Autodesk Inventor part; units mm, degrees
ref_plane "Work Plane1" through (0, 0, -15) normal (0, 0, 1) x (1, 0, 0)
ref_plane "YZ Plane" through (0, 0, 0) normal (1, 0, 0) x (0, 1, 0)
ref_plane "XZ Plane" through (0, 0, 0) normal (0, 1, 0) x (-1, 0, 0)
sketch "Sketch1" plane through (0, 0, 0) normal (0, 0, 1) x (1, 0, 0)
  line L0 (0, 0) -> (25, 0)
  line L1 (25, 0) -> (25, 40)
  line L2 (25, 40) -> (0, 40)
  line L3 (0, 40) -> (0, 0)
  dimension "d1" = 25
  dimension "d2" = 40
  dimension "d3" = 25
extrude "Extrusion1" add sketch "Sketch1" against normal blind 30
sketch "Sketch2" plane through (25, 0, 0) normal (1, 0, 0) x (0, 0, -1)
  line L0 (0, 0) -> (30, 0)
  circle A0 centre (15, 6.56) radius 2.46
extrude "Extrusion2" cut sketch "Sketch2" against normal blind 30
sketch "Sketch3" plane through (0, 0, 0) normal (-1, 0, 0) x (0, 0, 1)
  line L0 (0, 0) -> (-30, 0)
  line L1 (-25.05, 0) -> (-4.95, 0)
  line L2 (-4.95, 0) -> (-4.95, 33.12)
  line L3 (-4.95, 33.12) -> (-25.05, 33.12)
  line L4 (-25.05, 33.12) -> (-25.05, 0)
  dimension "d11" = 20.1
extrude "Extrusion3" cut sketch "Sketch3" against normal blind 20
sketch "Sketch4" plane through (0, 0, 0) normal (0, -1, 0) x (1, 0, 0)
  line L0 (20, -4.95) -> (20, -25.05)
  line L1 (20, -15) -> (25, -15)
  line L2 (25, 0) -> (25, -30)
  line L3 (20, -8.025) -> (25, -8.025)
  line L4 (25, -8.025) -> (25, -21.975)
  line L5 (25, -21.975) -> (20, -21.975)
  line L6 (20, -21.975) -> (20, -8.025)
  line L7 (20, -8.025) -> (25, -21.975) construction
  line L8 (25, -8.025) -> (20, -21.975) construction
  line L9 (25, -12.54) -> (25, -17.46)
  point P0 (0, 0)
  point P1 (22.5, -15)
  dimension "d14" = 13.95
extrude "Extrusion4" add sketch "Sketch4" along normal blind 15
sketch "Sketch5" plane through (20, 0, 0) normal (-1, 0, 0) x (0, 0, 1)
  circle A0 centre (-15, 6.56) radius 2.46
  circle A1 centre (-15, 6.56) radius 4.7025
  circle A2 centre (-15, 6.56) radius 2.46
  circle A3 centre (-15, 6.56) radius 2.46
  point P0 (0, 0)
  dimension "d17" = 9.405
extrude "Extrusion5" cut sketch "Sketch5" against normal blind 2.1
sketch "Sketch6" plane through (25, 0, 0) normal (1, 0, 0) x (0, 0, -1)
  circle A0 centre (15, 6.56) radius 4.7025
  line L0 (15, 6.56) -> (15, 23.56)
  circle A1 centre (15, 23.56) radius 2.46
  point P0 (0, 0)
  dimension "d20" = 17
  dimension "d21" = 4.92
extrude "Extrusion6" cut sketch "Sketch6" against normal blind 10 contours A1
sketch "Sketch7" plane through (20, 0, 0) normal (-1, 0, 0) x (0, 0, 1)
  circle A0 centre (-15, 23.56) radius 2.46
  circle A1 centre (-15, 23.56) radius 4.7025
  point P0 (0, 0)
  dimension "d24" = 9.405
extrude "Extrusion7" cut sketch "Sketch7" against normal blind 2.1
sketch "Sketch9" plane through (25, 0, 0) normal (1, 0, 0) x (0, 0, -1)
  circle A0 centre (15, 6.56) radius 2.46
  circle A1 centre (15, 6.56) radius 2.46
  circle A2 centre (15, 23.56) radius 2.46
  circle A3 centre (15, 23.56) radius 2.46
  line L0 (30, 40) -> (30, 0)
  line L1 (30, 0) -> (30, 40)
  line L2 (30, 40) -> (0, 40)
  line L3 (0, 40) -> (0, 0)
  line L4 (0, 0) -> (8.025, 0)
  line L5 (21.975, 0) -> (21.975, -15)
  line L6 (21.975, -15) -> (8.025, -15)
  line L7 (8.025, -15) -> (8.025, 0)
  line L8 (0, 0) -> (8.025, 0)
  line L9 (21.975, 0) -> (30, 0)
extrude "Extrusion8" add sketch "Sketch9" along normal blind 5
sketch "Sketch10" plane through (0, 40, 0) normal (0, 1, 0) x (1, 0, 0)
  line L0 (0, 30) -> (30, 30)
  line L1 (30, 0) -> (0, 0)
  line L2 (0, 30) -> (30, 30)
  line L3 (30, 30) -> (30, 0)
  line L4 (30, 0) -> (0, 0)
  line L5 (0, 0) -> (0, 30)
extrude "Extrusion9" add sketch "Sketch10" along normal blind 30
sketch "Sketch12" plane through (30, 0, 0) normal (1, 0, 0) x (0, 0, -1)
  circle A0 centre (15, 6.56) radius 2.46
  line L0 (15, 6.56) -> (15, 15.06)
  circle A1 centre (15, 15.06) radius 2.525
  point P0 (0, 0)
  dimension "d31" = 8.5
  dimension "d33" = 5.05
extrude "Extrusion10" cut sketch "Sketch12" against normal blind 30 contours A1
sketch "Sketch14" plane through (0, 0, 0) normal (0, 0, 1) x (1, 0, 0)
  line L0 (30, 70) -> (0, 70)
  line L1 (0, 100) -> (-8, 100)
  line L2 (30, 0) -> (30, 70)
  line L3 (30, 118) -> (30, 70)
  line L4 (30, 105) -> (30, 100)
  line L5 (0, 70) -> (30, 70)
  line L6 (0, 70) -> (0, 100)
  line L7 (15, 136) -> (30, 118)
  line L8 (-8, 136) -> (15, 136)
  line L9 (-8, 100) -> (-8, 136)
  point P0 (0, 0)
  dimension "d47" = 30
extrude "Extrusion12" add sketch "Sketch14" against normal blind 30
sketch "Sketch15" plane through (0, 0, -25.05) normal (-1, 0, 0) x (0, 0, 1)
  line L0 (0, 33.12) -> (20.1, 33.12)
  line L1 (20.1, 33.12) -> (20.1, 0)
  line L2 (0, 33.12) -> (20.1, 33.12)
  line L3 (20.1, 33.12) -> (20.1, 31.1)
  line L4 (20.1, 31.1) -> (0, 31.1)
  line L5 (0, 31.1) -> (0, 33.12)
  point P0 (25.05, 0)
  dimension "d57" = 2.02
extrude "Extrusion13" add sketch "Sketch15" against normal blind 20
sketch "Sketch23" plane through (0, 0, 0) normal (0, 0, 1) x (1, 0, 0)
  line L0 (0, 100) -> (-8, 100)
  line L1 (-8, 136) -> (15, 136)
  line L2 (-8, 136) -> (15, 136)
  line L3 (30, 118) -> (15, 136)
  line L4 (15, 136) -> (30, 118)
  line L5 (30, 118) -> (30, 93)
  line L6 (30, 0) -> (30, 118)
  line L7 (30, 93) -> (0, 93)
  line L8 (0, 93) -> (0, 100)
  line L9 (-8, 100) -> (0, 100)
  line L10 (15, 136) -> (-8, 136)
  line L11 (-8, 136) -> (-8, 100)
  point P0 (0, 0)
  point P1 (-2, 102)
  point P2 (4, 118)
  point P3 (-2, 134)
  dimension "d85" = 25
extrude "Extrusion14" add sketch "Sketch23" along normal blind 15
ref_plane "Work Plane1" through (0, 0, -15) normal (0, 0, 1) x (1, 0, 0)
mirror "Mirror1" about plane through (0, 0, -15) normal (0, 0, 1) of "Extrusion14"
sketch "Sketch28" plane through (-8, 136, 15) normal (0, 1, 0) x (1, 0, 0)
  line L0 (0, 60) -> (0, 0)
  line L1 (0, 30) -> (0, 5)
  line L2 (0, 5) -> (5, 5)
  line L3 (5, 5) -> (5, 55)
  line L4 (5, 55) -> (0, 55)
  line L5 (0, 55) -> (0, 30)
  line L6 (0, 55) -> (5, 30)
  line L7 (5, 30) -> (0, 5)
  point P0 (8, 15)
  dimension "d100" = 25
  dimension "d101" = 5
  dimension "d102" = 50
extrude "Extrusion17" cut sketch "Sketch28" against normal through all contours L6 L7 L0
properties part number "orien_b_45mm"
For this review, take the finished solid that the model builds, in its own axes (mm). A direction names the side the tool comes from. Coordinates: 2 decimals unless noted, no trailing zeros. Order: outer loops, then holes, each group sorted by start corner. A loop starts at its lowest first (then second) coordinate and runs counter-clockwise, first axis right, second up. Notation, with made-up numbers: (-25, 80.5) -> (-4, 80.5) arc R35 cw to (-4, 119.5) -> close; hole circle Ø5 at (62, 83.25). An arc over 180 degrees is marked (long way). Answer as CSV lines item,"result".
Q1. For faces 5 (the face through (10, 16, -25.05)), 6 (the face through (15, 47, 0)), 7 (the face through (21.035, 7.973, -10.515)), 8 (the face through (-2, 100, -15)), 9 (the face through (15, 47, -30)), list the 3-axis set-ups (+Z, -Z, +X, -X, +Y, -Y) from which the entire face can be reached by the end or side of a thin tool; tool diameter is ignored.
Model answer:
face 5,"-X, -Y"
face 6,"+Z, +X, -X, -Y"
face 7,"-X"
face 8,"+Z, -Z, -X, -Y"
face 9,"-Z, +X, -X, -Y"
Q2. Wall thickness on line 1 along Z through (x, y) = (3.5, 9); line 2 along Y through (x, z) = (27, -15) (3 decimals); line 3 along Y through (x, z) = (25, -15) (3 decimals): over which ranges is each line inside the solid? List them lowest first. Write a range as [from, to].
Model answer:
line 1,"z = [-30, -25.05], [-4.95, 0]"
line 2,"y = [-15, 4.1], [9.02, 12.535], [17.585, 21.1], [26.02, 121.6]"
line 3,"y = [-15, 4.1], [9.02, 12.535], [17.585, 21.1], [26.02, 124]"
Q3. We need section A-A (y = 23.56). State the section outline as (x, z) points, plus the area to 3 significant figures.
Model answer:
outline,"(0, -30) -> (30, -30) -> (30, -17.46) -> (22.1, -17.46) -> (22.1, -19.7) -> (20, -19.7) -> (20, -25.05) -> (0, -25.05) -> close; (0, -4.95) -> (20, -4.95) -> (20, -10.3) -> (22.1, -10.3) -> (22.1, -12.54) -> (30, -12.54) -> (30, 0) -> (0, 0) -> close"
area,"439 mm2"
Q4. We need section D-D (x = 18.5). State the section outline as (y, z) points.
Model answer:
outline,"(0, -30) -> (93, -30) -> (93, -45) -> (131.8, -45) -> (131.8, 15) -> (93, 15) -> (93, 0) -> (0, 0) -> (0, -4.95) -> (31.1, -4.95) -> (31.1, -25.05) -> (0, -25.05) -> close"
Q5. We need section B-B (x = 26). State the section outline as (y, z) points (3 decimals).
Model answer:
outline,"(-15, -21.975) -> (0, -21.975) -> (0, -30) -> (93, -30) -> (93, -45) -> (122.8, -45) -> (122.8, 15) -> (93, 15) -> (93, 0) -> (0, 0) -> (0, -8.025) -> (-15, -8.025) -> close; hole circle Ø4.92 at (6.56, -15); hole circle Ø5.05 at (15.06, -15); hole circle Ø4.92 at (23.56, -15)"
Q6. We need section C-C (z = 7.5). State the section outline as (x, y) points.
Model answer:
outline,"(-7.5, 100) -> (0, 100) -> (0, 93) -> (30, 93) -> (30, 118) -> (15, 136) -> (-7.5, 136) -> close"
Q7. Draft analysis for pull direction Y (two halves, no side actions). For faces 1 (the face through (22.395, 127.126, -14.58)), 2 (the face through (15, 0, -3)), 3 (the face through (25.995, 7.502, -17.272)), 4 (the face through (20, 8, -20)), state which applies: released by +Y, released by -Y, zero draft, split by the parting line, or undercut.
Model answer:
face 1,"released by +Y"
face 2,"released by -Y"
face 3,"undercut"
face 4,"zero draft"
Q8. Clearance check with flat-ended pins moving along their axes: pin 1 Ø10 at (y, z) = (13.5, -19) entering from -X; pin 2 Ø8 at (x, y) = (9.5, 7) entering from +Z; pin 3 Ø3 at (x, y) = (26, -6) entering from -Z (3 decimals); pin 4 Ø4 at (y, z) = (15.06, -15) entering from +X. State where each tip first meets the part, or that it passes through.
Model answer:
pin 1,"stops at x = 20"
pin 2,"stops at z = 0"
pin 3,"stops at z = -21.975"
pin 4,"passes through"
